Job drawing, mm, ordinate dimensions from the low corner. One solid piece. Give positions to 0.01 mm unless a question says otherwise; leave off trailing zeros. Order: outer loops, then holes, each group sorted by start corner. A loop starts at its lowest first (then second) coordinate and runs counter-clockwise, first axis right, second up. Notation, with made-up numbers: M 60,74 L 91,74 A27 ccw 91,100 Z; hole C 4,-12.75 d6. An arc over 180 degrees is marked long. Use CSV: the item, a comma, the result in double quotes. Start each with the question number.
Item 1: Pin check, flat tips, straight feed: P1, Ø2.5, axis at x = 41, z = 15, coming from the -Y side; P2, Ø1.5, axis at y = 2, z = 26, coming from the +X side; P3, Ø4, axis at x = 41, z = 115, coming from the -Y side; P4, Ø0.9, axis at y = 2, z = 40, coming from the -X side. Stop position of each tip, or through.
Item 2: Band-saw the part on A-A on z = 82.25. Write the cut outline in (x, y), plus the area to 3 significant figures.
Item 3: Band-saw the part on C-C on z = 15. Write the cut outline in (x, y), plus the area to 3 significant figures.
Item 4: Band-saw the part on D-D on z = 64. Write the cut outline in (x, y).
Item 5: Wall check: line 1 along X through (y, z) = (4.4, 75); line 2 along X through (y, z) = (5.7, 135); line 3 along X through (y, z) = (3.95, 82.25). Give the ranges that are in metal, low to high.
Item 6: Band-saw the part on B-B on x = 25. Write the cut outline in (y, z).
Item 7: Two-plate mould, pull along Z, no slides. Class the marked faces 1 and 2: pulls with the +Z half, pulls with the -Z half, needs draft (parallel to the pull), parting line crosses it, or undercut.
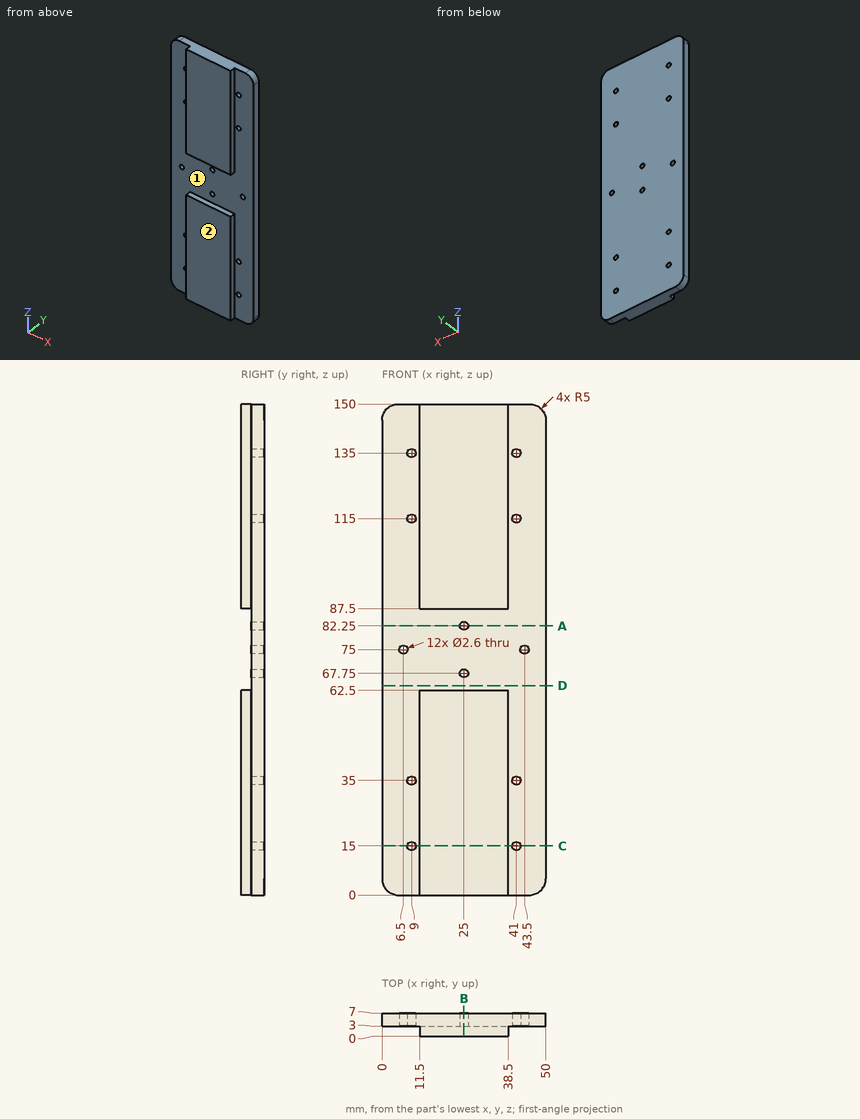
Model answer:
1,P1,"passes through"
1,P2,"stops at x = 38.5"
1,P3,"stops at y = 3"
1,P4,"stops at x = 11.5"
2,outline,"M 0,3 L 23.7,3 L 23.7,7 L 0,7 Z; M 26.3,3 L 50,3 L 50,7 L 26.3,7 Z"
2,area,"190 mm^2"
3,outline,"M 0,3 L 7.7,3 L 7.7,7 L 0,7 Z; M 10.3,3 L 11.5,3 L 11.5,0 L 38.5,0 L 38.5,3 L 39.7,3 L 39.7,7 L 10.3,7 Z; M 42.3,3 L 50,3 L 50,7 L 42.3,7 Z"
3,area,"260 mm^2"
4,outline,"M 0,3 L 50,3 L 50,7 L 0,7 Z"
5,line 1,"x = 0 to 5.2, 7.8 to 42.2, 44.8 to 50"
5,line 2,"x = 0 to 7.7, 10.3 to 39.7, 42.3 to 50"
5,line 3,"x = 0 to 23.7, 26.3 to 50"
6,outline,"M 0,0 L 7,0 L 7,66.45 L 3,66.45 L 3,62.5 L 0,62.5 Z; M 0,87.5 L 3,87.5 L 3,83.55 L 7,83.55 L 7,150 L 0,150 Z; M 3,69.05 L 7,69.05 L 7,80.95 L 3,80.95 Z"
7,face 1,"undercut"
7,face 2,"needs draft"
